Geometry check sheet. Reference: drawing and pictorial views, mm from the part's lowest x, y, z. Round coordinates to 2 decimals unless told otherwise and drop trailing zeros. Write each loop counter-clockwise with the first axis right and the second up, starting at its lowest first coordinate (ties: lowest second). Pieces come first, ordered by that corner, then holes. Notation, with made-up numbers: M -8,-37.5 L 51,-37.5 A18 ccw 51,-26.5 Z; hole C -21,-36.75 d2. An arc over 180 degrees is marked long. Answer in a Markdown table with one row per item.
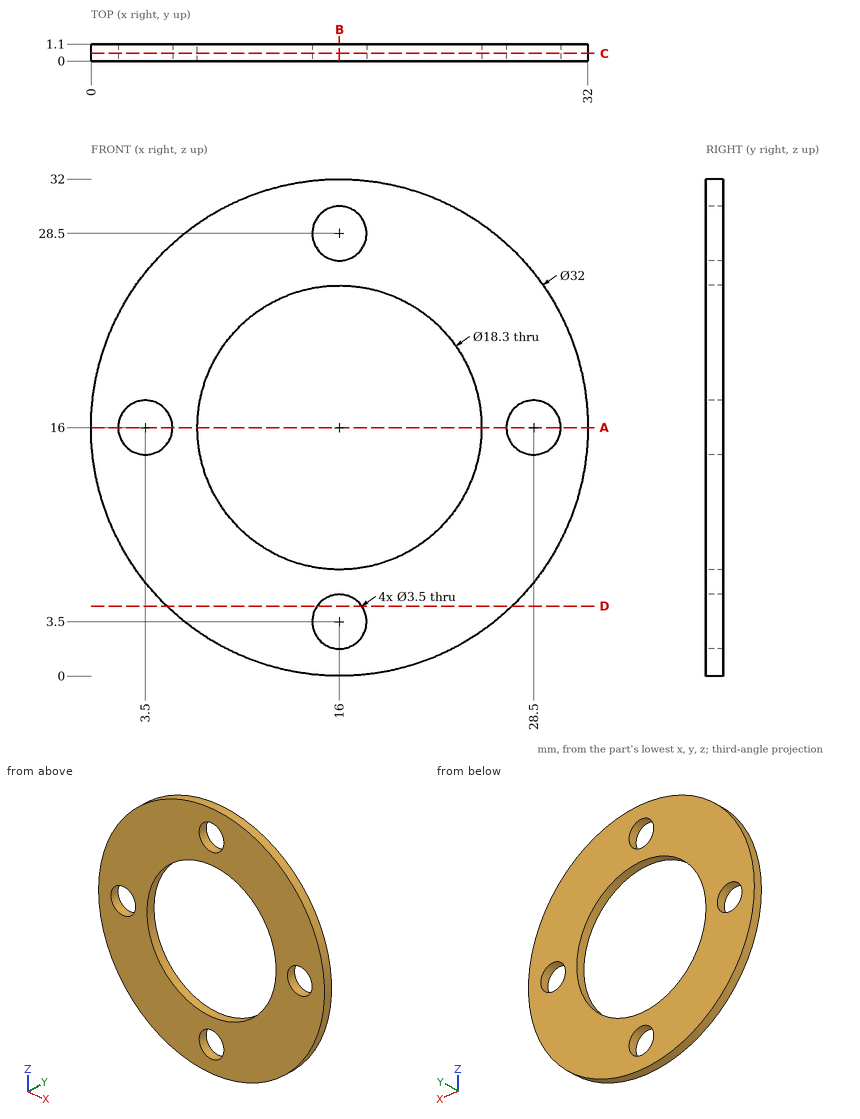
1. Section check D-D, the plane z = 4.5. Record the cut outline in (x, y).
Found:
| item | result |
|---|---|
| outline | M 4.88,0 L 14.56,0 L 14.56,1.1 L 4.88,1.1 Z; M 17.44,0 L 27.12,0 L 27.12,1.1 L 17.44,1.1 Z |
2. Section check B-B, the plane x = 16. Record the cut outline in (y, z), and give its area (3 significant figures).
Found:
| item | result |
|---|---|
| outline | M 0,0 L 1.1,0 L 1.1,1.75 L 0,1.75 Z; M 0,5.25 L 1.1,5.25 L 1.1,6.85 L 0,6.85 Z; M 0,25.15 L 1.1,25.15 L 1.1,26.75 L 0,26.75 Z; M 0,30.25 L 1.1,30.25 L 1.1,32 L 0,32 Z |
| area | 7.37 mm2 |
3. Scan lines: L1, parallel to Z at x = 16, y = 0.9; L2, parallel to Z at x = 15, y = 0.6; L3, parallel to X at y = 0.8, z = 10. Record each from-to range of solid material in increasing order.
Found:
| item | result |
|---|---|
| L1 | z = 0 to 1.75, 5.25 to 6.85, 25.15 to 26.75, 30.25 to 32 |
| L2 | z = 0.03 to 2.06, 4.94 to 6.9, 25.1 to 27.06, 29.94 to 31.97 |
| L3 | x = 1.17 to 9.09, 22.91 to 30.83 |
4. Go/stop test with a flat-tipped pin: pin 1 (1.5 mm diameter, centred on x = 24, z = 15.5, fed in from -Y). Record where the tip stops, or that it passes through.
Found:
| item | result |
|---|---|
| pin 1 | passes through |
5. Section check C-C, the plane y = 0.5. Record the cut outline in (x, z).
Found:
| item | result |
|---|---|
| outline | C 16,16 d32; hole C 3.5,16 d3.5; hole C 16,16 d18.3; hole C 16,3.5 d3.5; hole C 16,28.5 d3.5; hole C 28.5,16 d3.5 |
6. Section check A-A, the plane z = 16. Record the cut outline in (x, y).
Found:
| item | result |
|---|---|
| outline | M 0,0 L 1.75,0 L 1.75,1.1 L 0,1.1 Z; M 5.25,0 L 6.85,0 L 6.85,1.1 L 5.25,1.1 Z; M 25.15,0 L 26.75,0 L 26.75,1.1 L 25.15,1.1 Z; M 30.25,0 L 32,0 L 32,1.1 L 30.25,1.1 Z |
